```python
from build123d import *

# Parameters (mm, degrees)
F0_W      = 182.88
F0_H      = 182.88
F1_DEPTH  = 231.14
F2_T      = -2.54
F3_W      = 182.88
F3_H      = 182.88
F4_DEPTH  = 2.54
F6_DEPTH  = 2.54
F8_DEPTH  = 5.08
F10_DEPTH = 1.27


with BuildPart() as f1:
    # F0 (on Top) → F1 (new body)
    with BuildSketch(Plane.XY):
        Rectangle(F0_W, F0_H)
    extrude(amount=F1_DEPTH)

    # F2
    f2_openings = [f1.faces().sort_by_distance(p)[0] for p in [
        (0, 0, 231.14),
    ]]
    offset(amount=F2_T, openings=f2_openings)

    # F3 (on face) → F4 (join)
    with BuildSketch(Plane.XY.offset(231.14)):
        Rectangle(F3_W, F3_H)
    extrude(amount=F4_DEPTH)

    # F5 (on face) → F6 (join)
    with BuildSketch(Plane.XY.offset(233.68)):
        with BuildLine():
            Line((91.44, -91.44), (91.44, 91.44))
            Line((91.44, 91.44), (-68.0558882158, 28.342725541))
            ThreePointArc((-68.0558882158, 28.342725541), (-87.3233814083, 0), (-68.0558882158, -28.342725541))
            Line((-68.0558882158, -28.342725541), (91.44, -91.44))
        make_face()
    extrude(amount=F6_DEPTH)

    # F7 (on face) → F8 (join)
    with BuildSketch(Plane.XY.offset(233.68)):
        with BuildLine():
            Line((68.0558882158, 28.342725541), (-91.44, 91.44))
            Line((-91.44, 91.44), (-91.44, -91.44))
            Line((-91.44, -91.44), (68.0558882158, -28.342725541))
            ThreePointArc((68.0558882158, -28.342725541), (87.3233814083, 0), (68.0558882158, 28.342725541))
        make_face()
    extrude(amount=F8_DEPTH)

    # F9 (on Front) → F10 (join, symmetric)
    with BuildSketch(Plane.XZ):
        with BuildLine():
            Line((83.2395926118, 236.8696480989), (83.2395926118, 238.76))
            ThreePointArc((83.2395926118, 238.76), (-0.1585371792, 294.2423028387), (-83.5566669703, 238.76))
            Line((-83.5566669703, 238.76), (-83.6300104856, 236.8696480989))
            Line((-83.6300104856, 236.8696480989), (83.2395926118, 236.8696480989))
        make_face()
        with BuildLine():
            ThreePointArc((-54.5130875391, 254.6497191946), (0, 281.0305954441), (54.5130875391, 254.6497191946))
            Line((54.5130875391, 254.6497191946), (45.1730415225, 241.5446043015))
            Line((45.1730415225, 241.5446043015), (-45.6402897835, 241.5446043015))
            Line((-45.6402897835, 241.5446043015), (-54.5130875391, 254.6497191946))
        make_face(mode=Mode.SUBTRACT)
    extrude(amount=F10_DEPTH, both=True)


solid = f1.part
```
Geometry check sheet. Reference: the model listing, model coordinates, mm. A direction names the side the tool comes from. Coordinates: 2 decimals unless noted, no trailing zeros. Order: outer loops, then holes, each group sorted by start corner. A loop starts at its lowest first (then second) coordinate and runs counter-clockwise, first axis right, second up. Notation, with made-up numbers: (-26, 34.25) - (2, 34.25) arc R21 cw to (2, 72.25) - close; hole circle Ø6 at (29.5, -10.5). An arc over 180 degrees is marked (long way). Use one line per item in the form item = value.
1. Section check C-C (y = -76.5). Record the boundary of the cut face in (x, z) (3 decimals), then the cut area to 3 significant figures.
Here are the results:
outline = (-91.44, 0) - (91.44, 0) - (91.44, 236.22) - (53.675, 236.22) - (53.675, 233.68) - (-53.675, 233.68) - (-53.675, 238.76) - (-91.44, 238.76) - close; hole (-88.9, 2.54) - (88.9, 2.54) - (88.9, 231.14) - (-88.9, 231.14) - close
area = 2,380 mm²
2. Section check D-D (x = 71.5). Record the boundary of the cut face in (y, z), then the cut area to 3 significant figures.
Here are the results:
outline = (-91.44, 0) - (91.44, 0) - (91.44, 233.68) - (83.55, 233.68) - (83.55, 236.22) - (26.72, 236.22) - (26.72, 238.76) - (1.27, 238.76) - (1.27, 258.97) - (-1.27, 258.97) - (-1.27, 238.76) - (-26.72, 238.76) - (-26.72, 236.22) - (-83.55, 236.22) - (-83.55, 233.68) - (-91.44, 233.68) - close; hole (-88.9, 2.54) - (88.9, 2.54) - (88.9, 231.14) - (-88.9, 231.14) - close
area = 2,700 mm²
3. Gauge pin test, flat ends, axial feed: pin 1 (0.8 mm diameter, centred on x = 11.5, y = -0.5, fed in from +Z); pin 2 (8 mm diameter, centred on x = -64.5, y = -66.5, fed in from +Z); pin 3 (5 mm diameter, centred on x = -48.5, y = -45, fed in from -Z). Record the tip position at first contact, or that the pin passes through.
Here are the results:
pin_1 = 293.54
pin_2 = 238.76
pin_3 = 0
4. Access from +Z, -Z, +X, -X, +Y, -Y to the whole of each face (thin tool, end or side, straight path). Record for faces 4 (the face through (49.91, -0.02, 248.19)), 5 (the face through (-1, 1.27, 285)), 6 (the face through (45.08, -73.1, 234.93)), 7 (the face through (88.9, -1, 115)), 8 (the face through (-28.3, 66.46, 236.75)).
Here are the results:
face_4 = +Y, -Y
face_5 = +Z, +X, -X, +Y
face_6 = +Z, -Y
face_7 = none
face_8 = +Z, +Y
5. Section check B-B (z = 174). Record the boundary of the cut face in (x, y), then the cut area to 3 significant figures.
Here are the results:
outline = (-91.44, -91.44) - (91.44, -91.44) - (91.44, 91.44) - (-91.44, 91.44) - close; hole (-88.9, -88.9) - (88.9, -88.9) - (88.9, 88.9) - (-88.9, 88.9) - close
area = 1,830 mm²
6. Section check A-A (x = 8). Record the boundary of the cut face in (y, z).
Here are the results:
outline = (-91.44, 0) - (91.44, 0) - (91.44, 233.68) - (58.43, 233.68) - (58.43, 236.22) - (52.1, 236.22) - (52.1, 238.76) - (1.27, 238.76) - (1.27, 241.54) - (-1.27, 241.54) - (-1.27, 238.76) - (-52.1, 238.76) - (-52.1, 236.22) - (-58.43, 236.22) - (-58.43, 233.68) - (-91.44, 233.68) - close; (-1.27, 280.57) - (1.27, 280.57) - (1.27, 293.87) - (-1.27, 293.87) - close; hole (-88.9, 2.54) - (88.9, 2.54) - (88.9, 231.14) - (-88.9, 231.14) - close
7. Scan lines: line 1 (Z direction, x = 63, y = 77.5); line 2 (X direction, y = -26.5, z = 68). Record each from-to range of solid material in increasing order.
Here are the results:
line_1 = 0 to 2.54, 231.14 to 236.22
line_2 = -91.44 to -88.9, 88.9 to 91.44
8. Draft check along Z on faces 1 (the face through (-23, -19, 238.76)), 2 (the face through (-1, 1, 2.54)), 3 (the face through (-30.53, -67.344, 236.749)). Enter one of: pulls with the +Z half, pulls with the -Z half, needs draft (parallel to the pull), parting line crosses it, or undercut.
Here are the results:
face_1 = pulls with the +Z half
face_2 = undercut
face_3 = needs draft
